Answer from the drawing. Dimensions are ordinates in mm from the lowest x, y and z of the part. A direction names the side the tool comes from. Round coordinates to 2 decimals unless told otherwise and drop trailing zeros. Write each loop counter-clockwise with the first axis right and the second up, starting at its lowest first coordinate (ties: lowest second). Pieces come first, ordered by that corner, then holes. Notation, with made-up numbers: (-31.5, 42) - (-16.5, 42) arc R10 cw to (-16.5, 57) - close; hole circle Ø4 at (45.25, 66.5). An arc over 180 degrees is marked (long way). Answer in a Markdown table with one row per item.
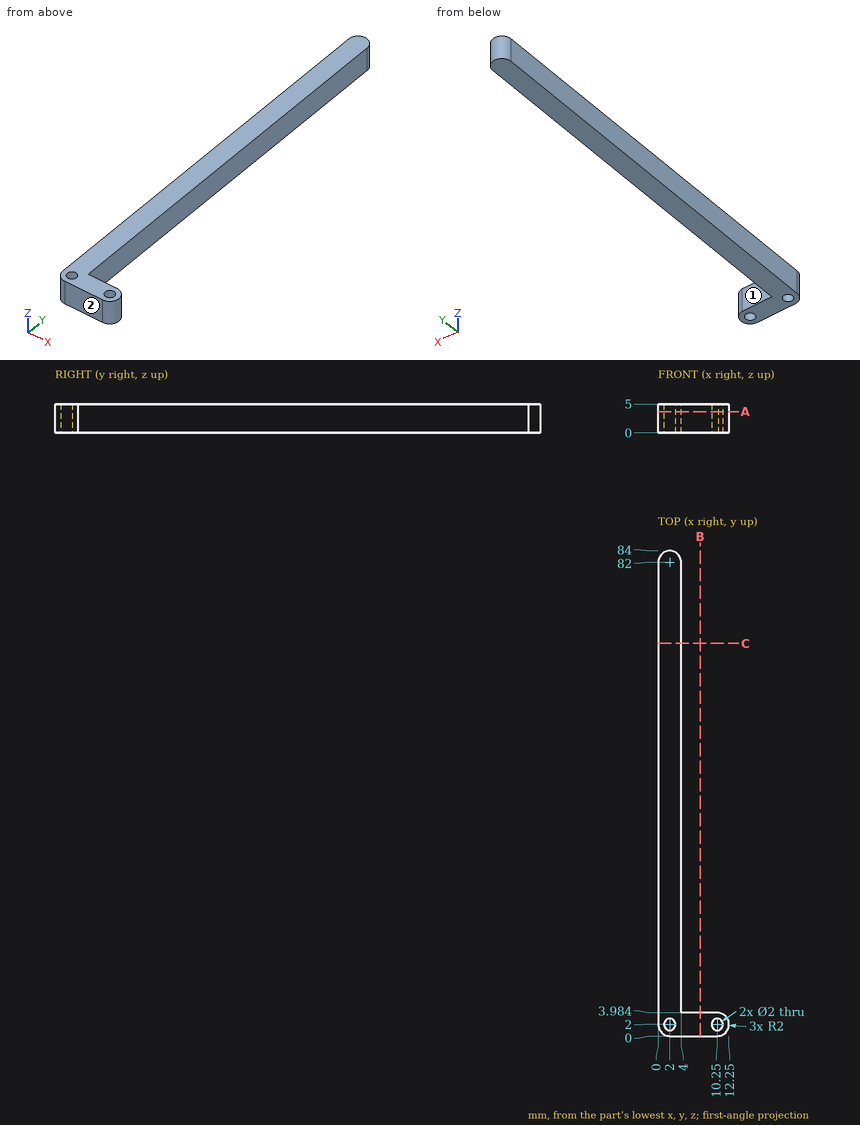
(1) Section C-C (y = 68) is taken. Give the vertices of the cut face in (x, z), and give its area (3 significant figures).
Checked values:
| item | result |
|---|---|
| outline | (0, 0) - (4, 0) - (4, 5) - (0, 5) - close |
| area | 20.0 mm2 |
(2) Section B-B (x = 7.25) is taken. Give the vertices of the cut face in (y, z), and give its area (3 significant figures).
Checked values:
| item | result |
|---|---|
| outline | (0, 0) - (3.98, 0) - (3.98, 5) - (0, 5) - close |
| area | 19.9 mm2 |
(3) Flat-ended cylindrical pins translate along their axes: pin 1 (1.5 mm diameter, centred on y = 48.5, z = 3.5, fed in from +X); pin 2 (1.5 mm diameter, centred on x = 6, z = 3.5, fed in from +Y). Find the tip coordinate at first contact, or state that the pin passes through.
Checked values:
| item | result |
|---|---|
| pin 1 | stops at x = 4 |
| pin 2 | stops at y = 3.98 |
(4) Find the intervals of material crossed by line 1 (Y direction, x = 10.25, z = 2.2); line 2 (Y direction, x = 2, z = 1.75); line 3 (X direction, y = 26.5, z = 0.45), in increasing order.
Checked values:
| item | result |
|---|---|
| line 1 | y = 0 to 1, 3 to 3.98 |
| line 2 | y = 0 to 1, 3 to 84 |
| line 3 | x = 0 to 4 |
(5) Section A-A (z = 3.7) is taken. Give the vertices of the cut face in (x, y).
Checked values:
| item | result |
|---|---|
| outline | (0, 2) arc R2 ccw to (2, 0) - (10.25, 0) arc R2 ccw to (10.5, 3.98) - (4, 3.98) - (4, 81.98) arc R2 ccw (long way) to (0, 82) - close; hole circle Ø2 at (2, 2); hole circle Ø2 at (10.25, 2) |
(6) For the marked faces 1 and 2, determine the directions among +Z, -Z, +X, -X, +Y, -Y from which every point of the face is accessible in a straight line to the end or side of a thin tool.
Checked values:
| item | result |
|---|---|
| face 1 | +Z, -Z, +X, +Y |
| face 2 | +Z, -Z, +X, -X, -Y |
